For this review, take the finished solid that the model builds, in its own axes (mm). Face numbers are marked on the shaded views. A direction names the side the tool comes from. Coordinates: 2 decimals unless noted, no trailing zeros. Order: outer loops, then holes, each group sorted by start corner. A loop starts at its lowest first (then second) coordinate and runs counter-clockwise, first axis right, second up.
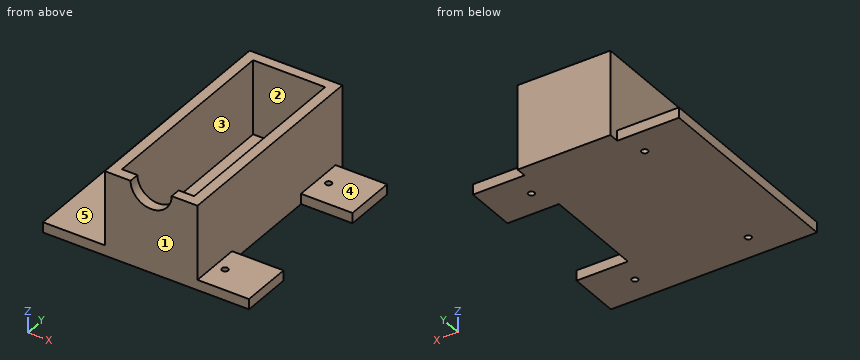
from build123d import *

# Parameters (mm, degrees)
F0_W      = 44.45
F0_H      = 45.72
F1_DEPTH  = 120.65
F2_T      = 6.35
F4_W      = 38.1
F4_H      = 6.35
F5_DEPTH  = 127
F6_W      = 31.75
F6_H      = 6.35
F7_DEPTH  = 38.1
F3_W      = 31.75
F3_H      = 6.35
F8_DEPTH  = 38.1
F10_D     = 3.81
F12_D     = 3.81
F14_D     = 3.81
F16_D     = 3.81
F18_D     = 25.4
F18_DEPTH = 15.1
F18_TIP   = 7.6309298617


with BuildPart() as f1:
    # F0 (on Front) → F1 (new body)
    with BuildSketch(Plane.XZ):
        with Locations((-22.225, 22.86)):
            Rectangle(F0_W, F0_H)
    extrude(amount=F1_DEPTH)

    # F2
    f2_openings = [f1.faces().sort_by_distance(p)[0] for p in [
        (-22.225, -60.325, 45.72),
    ]]
    offset(amount=F2_T, openings=f2_openings, kind=Kind.INTERSECTION)

    # F4 (on Front) → F5 (join)
    with BuildSketch(Plane.XZ):
        with Locations((-69.85, -3.175)):
            Rectangle(F4_W, F4_H)
    extrude(amount=F5_DEPTH)

    # F6 (on Right) → F7 (join)
    with BuildSketch(Plane.YZ):
        with Locations((-111.125, -3.175)):
            Rectangle(F6_W, F6_H)
    extrude(amount=F7_DEPTH)

    # F3 (on Right) → F8 (join)
    with BuildSketch(Plane.YZ):
        with Locations((-15.875, -3.175)):
            Rectangle(F3_W, F3_H)
    extrude(amount=F8_DEPTH)

    # F10 (through all)
    with Locations(Plane.XY):
        with Locations((-57.15, -111.125)):
            Hole(F10_D / 2)

    # F12 (through all)
    with Locations(Plane.XY):
        with Locations((-57.15, -15.875)):
            Hole(F12_D / 2)

    # F14 (through all)
    with Locations(Plane.XY):
        with Locations((12.7, -111.125)):
            Hole(F14_D / 2)

    # F16 (through all)
    with Locations(Plane.XY):
        with Locations((12.7, -15.875)):
            Hole(F16_D / 2)

    # F18
    with Locations(Plane.XZ.offset(127)):
        with Locations((-22.225, 45.72)):
            Hole(F18_D / 2, depth=F18_DEPTH)
            with Locations((0, 0, -(F18_DEPTH + F18_TIP / 2))):  # 118° drill point
                Cone(0, F18_D / 2, F18_TIP, mode=Mode.SUBTRACT)


solid = f1.part
1. Clearance check with flat-ended pins moving along their axes: pin 1 Ø23 at (y, z) = (-69, 23) entering from +X; pin 2 Ø7 at (x, z) = (-64, -3.5) entering from +Y; pin 3 Ø9.5 at (x, y) = (19, -20) entering from +Z; pin 4 Ø12 at (y, z) = (-8, 2.5) entering from -X. State where each tip first meets the part, or that it passes through.
Answer below:
pin 1: stops at x = 6.35
pin 2: stops at y = 0
pin 3: stops at z = 0
pin 4: stops at x = -88.9
2. Take a section at A-A, the plane x = -57.15. Give the boundary of the cut face in (y, z), plus the area to 3 significant figures.
Answer below:
outline: (-127, -6.35) - (-113.03, -6.35) - (-113.03, 0) - (-127, 0) - close; (-109.22, -6.35) - (-17.78, -6.35) - (-17.78, 0) - (-109.22, 0) - close; (-13.97, -6.35) - (0, -6.35) - (0, 0) - (-13.97, 0) - close
area: 758 mm2
3. Take a section at D-D, the plane z = 21.5. Give the boundary of the cut face in (x, y), plus the area to 3 significant figures.
Answer below:
outline: (-50.8, -127) - (6.35, -127) - (6.35, 6.35) - (-50.8, 6.35) - close; hole (-44.45, -120.65) - (0, -120.65) - (0, 0) - (-44.45, 0) - close
area: 2,260 mm2
4. Machinability: for the marked faces 3, 4 and 5, which of the approach directions +Z, -Z, +X, -X, +Y, -Y give a long, thin tool a straight path to every point of the face, cutting with its end or side? Answer none if there is none.
Answer below:
face 3: +Z
face 4: +Z, +X, +Y, -Y
face 5: +Z, -X, +Y, -Y
5. To check wall thickness, follow L1, parallel to Y at x = -57.15, z = -3.25; L2, parallel to X at y = -63, z = 6.5; L3, parallel to Y at x = -1, z = 29. State the ranges of each line that lie inside material, in increasing order.
Answer below:
L1: y = -127 to -113.03, -109.22 to -17.78, -13.97 to 0
L2: x = -50.8 to -44.45, 0 to 6.35
L3: y = -127 to -120.65, 0 to 6.35
6. Take a section at B-B, the plane x = 27. Give the boundary of the cut face in (y, z), plus the area to 3 significant figures.
Answer below:
outline: (-127, -6.35) - (-95.25, -6.35) - (-95.25, 0) - (-127, 0) - close; (-31.75, -6.35) - (0, -6.35) - (0, 0) - (-31.75, 0) - close
area: 403 mm2
7. Take a section at C-C, the plane y = -59.5. Give the boundary of the cut face in (x, z).
Answer below:
outline: (-88.9, -6.35) - (6.35, -6.35) - (6.35, 45.72) - (0, 45.72) - (0, 0) - (-44.45, 0) - (-44.45, 45.72) - (-50.8, 45.72) - (-50.8, 0) - (-88.9, 0) - close
8. The part is to be moulded in two halves that separate along X. For the marked faces 1 and 2, say which applies: +X half, -X half, draft (parallel to the pull), parting line (faces both ways), or undercut.
Answer below:
face 1: draft
face 2: undercut
